CAD build for the part. Positions are in the model's coordinates, mm. A direction names the side the tool comes from. Give positions to 0.01 mm unless a question says otherwise; leave off trailing zeros. Loops run counter-clockwise (first coordinate to the right, second up) from the corner with the lowest first, then second, coordinate; pieces in that order, holes last. Notation, with made-up numbers: (19.25, 57) - (37.25, 57) arc R21 cw to (37.25, 80) - close; hole circle Ø10 at (4.5, 2). An arc over 180 degrees is marked (long way). Return JSON: item names as keys, results as strings.
Autodesk Inventor part; units mm, degrees
ref_plane "YZ Plane" through (0, 0, 0) normal (1, 0, 0) x (0, 1, 0)
ref_plane "XZ Plane" through (0, 0, 0) normal (0, 1, 0) x (-1, 0, 0)
ref_plane "XY Plane" through (0, 0, 0) normal (0, 0, 1) x (1, 0, 0)
sketch "スケッチ1" plane through (0, 0, 0) normal (0, 0, 1) x (1, 0, 0)
  line L0 (0, 0) -> (15, 0)
  line L1 (15, 0) -> (15, 15)
  line L2 (15, 15) -> (0, 15)
  line L3 (0, 15) -> (0, 0)
  dimension "d0" = 15
  dimension "d1" = 15
extrude "押し出し1" add sketch "スケッチ1" along normal blind 50
sketch "スケッチ3" plane through (0, 0, 0) normal (0, 0, -1) x (-1, 0, 0)
  line L0 (0, 15) -> (0, 0)
  line L1 (0, 0) -> (-15, 0)
  line L2 (-15, 0) -> (-15, 15)
  line L3 (-15, 15) -> (0, 15)
  line L4 (0, 15) -> (0, 0)
  dimension "d21" = 15
  dimension "d22" = 15
extrude "押し出し2" add sketch "スケッチ3" along normal blind 135
sketch "スケッチ4" plane through (0, 15, 50) normal (0, 1, 0) x (1, 0, 0)
  line L0 (15, 0) -> (15, 185)
  line L1 (15, 185) -> (0, 185)
  line L2 (0, 185) -> (0, 105)
  line L3 (0, 105) -> (15, 105)
  line L4 (15, 105) -> (15, 185)
  point P0 (0, 50)
  dimension "d25" = 15
  dimension "d26" = 80
extrude "押し出し3" cut sketch "スケッチ4" against normal blind 135
sketch "スケッチ5" plane through (15, 15, -55) normal (0, 0, -1) x (-1, 0, 0)
  line L0 (15, 0) -> (15, -15)
  line L1 (0, -15) -> (0, 0)
  line L2 (15, -15) -> (0, -15)
  line L3 (0, -15) -> (0, 0)
  line L4 (0, 0) -> (15, 0)
  line L5 (15, 0) -> (15, -15)
extrude "押し出し4" add sketch "スケッチ5" along normal blind 15
sketch "スケッチ8" plane through (15, 0, 50) normal (1, 0, 0) x (0, 0, -1)
  line L0 (120, 15) -> (120, 0)
  line L1 (120, 15) -> (0, 15)
  point P0 (50, 0)
  point P1 (90, 7.5)
  point P2 (80, 7.5)
  point P3 (70, 7.5)
  dimension "d54" = 30
  dimension "d55" = 7.5
  dimension "d56" = 7.5
  dimension "d57" = 7.5
  dimension "d58" = 10
  dimension "d59" = 10
hole "穴4" at (15, 7.5, -40) at (15, 7.5, -30) at (15, 7.5, -20) direction (-1, 0, 0) diameter 3.2 end through all
sketch "スケッチ9" plane through (15, 0, 50) normal (1, 0, 0) x (0, 0, -1)
  line L0 (0, 0) -> (0, 15)
  line L1 (0, 0) -> (120, 0)
  point P0 (50, 0)
  point P1 (10, 7.5)
  point P2 (20, 7.5)
  dimension "d67" = 10
  dimension "d68" = 10
  dimension "d69" = 7.5
  dimension "d70" = 7.5
hole "穴5" at (15, 7.5, 40) at (15, 7.5, 30) direction (-1, 0, 0) diameter 3.2 end through all
sketch "スケッチ10" plane through (15, 15, -70) normal (0, 0, -1) x (-1, 0, 0)
  line L0 (15, 0) -> (0, 0)
  line L1 (15, -15) -> (0, -15)
  line L2 (0, -15) -> (0, 0)
  line L3 (0, 0) -> (15, 0)
  line L4 (15, 0) -> (15, -15)
extrude "押し出し5" cut sketch "スケッチ10" against normal blind 10
sketch "スケッチ11" plane through (0, 0, 50) normal (0, 0, 1) x (1, 0, 0)
  line L0 (1.5, 13.5) -> (13.5, 13.5)
  line L1 (13.5, 13.5) -> (13.5, 1.5)
  line L2 (13.5, 1.5) -> (1.5, 1.5)
  line L3 (1.5, 1.5) -> (1.5, 13.5)
  line L4 (15, 15) -> (0, 15)
  line L5 (0, 15) -> (0, 0)
  dimension "d80" = 12
  dimension "d81" = 12
  dimension "d82" = 1.5
  dimension "d83" = 1.5
extrude "押し出し6" cut sketch "スケッチ11" against normal blind 140
properties part number "射出_角柱6" material "アルミニウム 6061"
1. Which spindle directions (+Z, -Z, +X, -X, +Y, -Y) get a long thin tool onto all of the face, cutting with end or side? Do faces 4 (the face through (14.24, 9.06, -39.65)), 5 (the face through (8, 1.5, -4)). Say none if no direction does.
Values follow:
{"face 4": "+X, -X", "face 5": "+Z, -Z"}
2. Pull direction Y, two halves, no side cores. Call faces 1 (the face through (7, 0, -4)), 2 (the face through (15, 7, -4)), 3 (the face through (7, 13.5, -4)): +Y half, -Y half, draft (parallel to the pull), parting line (faces both ways), or undercut.
Values follow:
{"face 1": "-Y half", "face 2": "draft", "face 3": "undercut"}
3. Cut at A-A, the plane z = -37.5. Write the cut outline in (x, y), plus the area to 3 significant figures.
Values follow:
{"outline": "(0, 0) - (15, 0) - (15, 15) - (0, 15) - close; hole (1.5, 1.5) - (13.5, 1.5) - (13.5, 13.5) - (1.5, 13.5) - close", "area": "81.0 mm²"}
4. Cut at D-D, the plane z = 30. Write the cut outline in (x, y), plus the area to 3 significant figures.
Values follow:
{"outline": "(0, 0) - (15, 0) - (15, 5.9) - (13.5, 5.9) - (13.5, 1.5) - (1.5, 1.5) - (1.5, 5.9) - (0, 5.9) - close; (0, 9.1) - (1.5, 9.1) - (1.5, 13.5) - (13.5, 13.5) - (13.5, 9.1) - (15, 9.1) - (15, 15) - (0, 15) - close", "area": "71.4 mm²"}
5. Drill centre lines: probe 1 along Z at (x, y) = (0.4, 7.5); probe 2 along X at (y, z) = (12.25, -33). Where is each one in solid material? Low to high.
Values follow:
{"probe 1": "z = -60 to -41.6, -38.4 to -31.6, -28.4 to -21.6, -18.4 to 28.4, 31.6 to 38.4, 41.6 to 50", "probe 2": "x = 0 to 1.5, 13.5 to 15"}
6. Cut at B-B, the plane x = 12.25. Write the cut outline in (y, z), plus the area to 3 significant figures.
Values follow:
{"outline": "(0, -60) - (1.5, -60) - (1.5, 50) - (0, 50) - close; (13.5, -60) - (15, -60) - (15, 50) - (13.5, 50) - close", "area": "330 mm²"}
